from build123d import *

# Parameters (mm, degrees)
EXTRUDE_2_DEPTH     = 5
SKETCH_2_R          = 3.2
CUT_EXTRUDE_1_DEPTH = 5
SKETCH_4_W          = 36
SKETCH_4_H          = 25
EXTRUDE_3_DEPTH     = 30
FILLET_1_R          = 2.5
EXTRUDE_4_DEPTH     = 30
SKETCH_6_R          = 3.2
CUT_EXTRUDE_2_DEPTH = 36


with BuildPart() as part:
    # 스케치1 → 보스-돌출2 (new body)
    with BuildSketch(Plane(origin=(0, 0, 0), x_dir=(1, 0, 0), z_dir=(0, 1, 0))):
        with BuildLine():
            Line((-32.5, 37.5), (32.5, 37.5))
            ThreePointArc((32.5, 37.5), (36.035533906, 36.035533906), (37.5, 32.5))
            Line((37.5, 32.5), (37.5, -32.5))
            ThreePointArc((37.5, -32.5), (36.035533906, -36.035533906), (32.5, -37.5))
            Line((32.5, -37.5), (-32.5, -37.5))
            ThreePointArc((-32.5, -37.5), (-36.035533906, -36.035533906), (-37.5, -32.5))
            Line((-37.5, -32.5), (-37.5, 32.5))
            ThreePointArc((-37.5, 32.5), (-36.035533906, 36.035533906), (-32.5, 37.5))
        make_face()
    extrude(amount=EXTRUDE_2_DEPTH)

    # 스케치2 → 컷-돌출1 (cut)
    with BuildSketch(Plane(origin=(0, 5, 0), x_dir=(1, 0, 0), z_dir=(0, 1, 0))):
        with Locations((0, 25)):
            Circle(SKETCH_2_R)
        with Locations((-25, 25)):
            Circle(SKETCH_2_R)
        with Locations((-25, 0)):
            Circle(SKETCH_2_R)
        with Locations((-25, -25)):
            Circle(SKETCH_2_R)
        with Locations((0, -25)):
            Circle(SKETCH_2_R)
        with Locations((25, -25)):
            Circle(SKETCH_2_R)
        with Locations((25, 0)):
            Circle(SKETCH_2_R)
        with Locations((25, 25)):
            Circle(SKETCH_2_R)
    extrude(amount=-CUT_EXTRUDE_1_DEPTH, mode=Mode.SUBTRACT)

    # 스케치4 → 보스-돌출3 (add)
    with BuildSketch(Plane(origin=(0, 35, 0), x_dir=(-1, 0, 0), z_dir=(0, -1, 0))):
        with Locations((0, -6)):
            Rectangle(SKETCH_4_W, SKETCH_4_H)
    extrude(amount=EXTRUDE_3_DEPTH)

    # 필렛1
    fillet_1_edges = [part.edges().sort_by_distance(p)[0] for p in [
        (-18, 20, -6.5),
        (-18, 20, 18.5),
        (18, 20, 18.5),
        (18, 20, -6.5),
    ]]
    fillet(fillet_1_edges, radius=FILLET_1_R)

    # 스케치5 → 보스-돌출4 (add)
    with BuildSketch(Plane(origin=(0, 65, 0), x_dir=(-1, 0, 0), z_dir=(0, -1, 0))):
        with BuildLine():
            Line((18, -16), (18, 4))
            ThreePointArc((18, 4), (17.267766953, 5.767766953), (15.5, 6.5))
            Line((15.5, 6.5), (11.25, 6.5))
            Line((11.25, 6.5), (11.25, -18.5))
            Line((11.25, -18.5), (15.5, -18.5))
            ThreePointArc((15.5, -18.5), (17.267766953, -17.767766953), (18, -16))
        make_face()
        with BuildLine():
            Line((-18, -16), (-18, 4))
            ThreePointArc((-18, 4), (-17.267766953, 5.767766953), (-15.5, 6.5))
            Line((-15.5, 6.5), (-11.25, 6.5))
            Line((-11.25, 6.5), (-11.25, -18.5))
            Line((-11.25, -18.5), (-15.5, -18.5))
            ThreePointArc((-15.5, -18.5), (-17.267766953, -17.767766953), (-18, -16))
        make_face()
    extrude(amount=EXTRUDE_4_DEPTH)

    # 스케치6 → 컷-돌출2 (cut)
    with BuildSketch(Plane(origin=(18, 0, 0), x_dir=(0, 0, -1), z_dir=(1, 0, 0))):
        with Locations((-6, 57.5)):
            Circle(SKETCH_6_R)
        with Locations((-6, 42.5)):
            Circle(SKETCH_6_R)
    extrude(amount=-CUT_EXTRUDE_2_DEPTH, mode=Mode.SUBTRACT)


solid = part.part
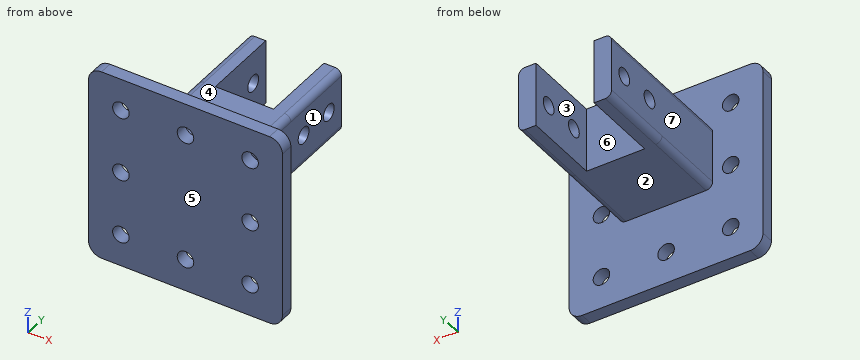
Source: CAD feature listing. Evaluate the final solid. Frame: model axes, mm. Face numbers are marked on the shaded views. A direction names the side the tool comes from. Give positions to 0.01 mm unless a question says otherwise; leave off trailing zeros. Write each loop counter-clockwise with the first axis right and the second up, starting at its lowest first coordinate (ties: lowest second). Pieces come first, ordered by that corner, then holes. Notation, with made-up numbers: (42, 63) - (52, 63) arc R17 ccw to (52, 72) - close; hole circle Ø7 at (-28.75, 65.5). An arc over 180 degrees is marked (long way). Write item = value, one per line. Start each with the question number.
Q1. Cut plane A-A, the plane x = 0. Return loops of the section in (y, z), then the cut area to 3 significant figures.
Q2. Draft query along X for the marked faces 1, 2 and 3. Return one class per face: +X half, -X half, draft (parallel to the pull), parting line (faces both ways), or undercut.
Q3. Cut plane D-D, the plane x = -25. Return loops of the section in (y, z).
Q4. Reachability of the marked faces 4, 5, 6 and 7 from +Z, -Z, +X, -X, +Y, -Y: full face, straight path, thin tool, end or side. Return the list, or none.
Q5. Cut plane B-B, the plane y = 42.5. Return loops of the section in (x, z).
Q6. Material intervals for probe 1 along X at (y, z) = (1.5, 0); probe 2 along Z at (x, y) = (25, 2), sorted ascending.
Q7. Cut plane C-C, the plane z = 25. Return loops of the section in (x, y), then the cut area to 3 significant figures.
Q8. Pin query (flat end, axial travel): pin 1 Ø1 at (x, y) = (11.5, 49) entering from +Z; pin 2 Ø1.5 at (y, z) = (13.5, 15.5) entering from +X; pin 3 Ø10 at (x, z) = (25, 0) entering from +Y; pin 4 Ø4 at (x, z) = (-25, 0) entering from -Y. Return the tip coordinate at first contact, or that it passes through.
Computed values:
q1.outline = (0, -37.5) - (5, -37.5) - (5, -28.2) - (0, -28.2) - close; (0, -21.8) - (5, -21.8) - (5, -6.5) - (35, -6.5) - (35, 18.5) - (5, 18.5) - (5, 21.8) - (0, 21.8) - close; (0, 28.2) - (5, 28.2) - (5, 37.5) - (0, 37.5) - close
q1.area = 1,060 mm²
q2.face_1 = +X half
q2.face_2 = draft
q2.face_3 = undercut
q3.outline = (0, -37.5) - (5, -37.5) - (5, -28.2) - (0, -28.2) - close; (0, -21.8) - (5, -21.8) - (5, -3.2) - (0, -3.2) - close; (0, 3.2) - (5, 3.2) - (5, 21.8) - (0, 21.8) - close; (0, 28.2) - (5, 28.2) - (5, 37.5) - (0, 37.5) - close
q4.face_4 = +Z, +X, -X, +Y
q4.face_5 = +Z, -Z, +X, -X, -Y
q4.face_6 = +Z, -Z, +Y
q4.face_7 = +Z, -Z, -X, +Y
q5.outline = (-18, -4) arc R2.5 ccw to (-15.5, -6.5) - (-11.25, -6.5) - (-11.25, 2.8) - (-18, 2.8) - close; (-18, 9.2) - (-11.25, 9.2) - (-11.25, 18.5) - (-15.5, 18.5) arc R2.5 ccw to (-18, 16) - close; (11.25, -6.5) - (15.5, -6.5) arc R2.5 ccw to (18, -4) - (18, 2.8) - (11.25, 2.8) - close; (11.25, 9.2) - (18, 9.2) - (18, 16) arc R2.5 ccw to (15.5, 18.5) - (11.25, 18.5) - close
q6.probe_1 = -37.5 to -28.2, -21.8 to 21.8, 28.2 to 37.5
q6.probe_2 = -37.5 to -28.2, -21.8 to -3.2, 3.2 to 21.8, 28.2 to 37.5
q7.outline = (-37.5, 0) - (-28.2, 0) - (-28.2, 5) - (-37.5, 5) - close; (-21.8, 0) - (-3.2, 0) - (-3.2, 5) - (-21.8, 5) - close; (3.2, 0) - (21.8, 0) - (21.8, 5) - (3.2, 5) - close; (28.2, 0) - (37.5, 0) - (37.5, 5) - (28.2, 5) - close
q7.area = 279 mm²
q8.pin_1 = 18.5
q8.pin_2 = 18
q8.pin_3 = 5
q8.pin_4 = through
